Can you work these out from the model? Positions are in its coordinate system, mm. A direction names the side the tool comes from. Coordinates: 2 decimals unless noted, no trailing zeros. Loops run counter-clockwise (first coordinate to the right, second up) from the corner with the lowest first, then second, coordinate; pieces in that order, holes last. Notation, with made-up numbers: (-0.75, 26.5) -> (20.25, 26.5) arc R14 ccw to (20.25, 40.5) -> close; hole circle Ø4 at (75.25, 13). An arc over 180 degrees is marked (long way). Put each result on its own line as item: value. Start each with the question number.
Item 1: We'd pull the mould along X, two halves only. Please class faces 1 (the flat face through (25.4, 614, -25)), 2 (the flat face through (2, 0, -27)), 3 (the flat face through (13, 614, -2.54)): pulls with the +X half, pulls with the -X half, needs draft (parallel to the pull), parting line crosses it, or undercut.
Item 2: Please list where these lines run through material, in increasing order: L1, parallel to Y at x = 1.5, z = -12.7; L2, parallel to Y at x = 1.45, z = -38.1; L3, parallel to X at y = 435, z = -26. Write a range as from..to.
Item 3: For faces 4 (the flat face through (2.54, 614, -25)), 5 (the flat face through (0, 614, -25)), which set-ups out of +Z, -Z, +X, -X, +Y, -Y let a thin tool reach every point of the face, with its end or its side?
Item 4: If we section it at A-A on y = 861: Please give me the cut outline in (x, z).
```python
from build123d import *

# Parameters (mm, degrees)
SKETCH1_W           = 25.4
SKETCH1_H           = 50.8
SKETCH1_W_2         = 20.32
SKETCH1_H_2         = 45.72
EXTRUDE_THIN1_DEPTH = 1244.6
SKETCH2_R           = 2.4892
CUT_EXTRUDE1_DEPTH  = 26.4
SKETCH3_R           = 2.5019
SKETCH3_R_2         = 2.4892
CUT_EXTRUDE2_DEPTH  = 26.4
SKETCH5_R           = 2.4892
CUT_EXTRUDE3_DEPTH  = 51.8
SKETCH6_R           = 3.175
CUT_EXTRUDE4_DEPTH  = 51.8
SKETCH7_R           = 3.175
CUT_EXTRUDE5_DEPTH  = 51.8


with BuildPart() as part:
    # Sketch1 → Extrude-Thin1 (new body)
    with BuildSketch(Plane(origin=(0, 0, 0), x_dir=(1, 0, 0), z_dir=(0, 1, 0))):
        with Locations((12.7, 25.4)):
            Rectangle(SKETCH1_W, SKETCH1_H)
        with Locations((12.7, 25.4)):
            Rectangle(SKETCH1_W_2, SKETCH1_H_2, mode=Mode.SUBTRACT)
    extrude(amount=EXTRUDE_THIN1_DEPTH)

    # Sketch2 → Cut-Extrude1 (cut, through all)
    with BuildSketch(Plane(origin=(25.4, 0, 0), x_dir=(0, 0, -1), z_dir=(1, 0, 0))):
        with Locations((25.4, 1200.15)):
            Circle(SKETCH2_R)
        with Locations((25.4, 1212.85)):
            Circle(SKETCH2_R)
    extrude(amount=-CUT_EXTRUDE1_DEPTH, mode=Mode.SUBTRACT)

    # Sketch3 → Cut-Extrude2 (cut, through all)
    with BuildSketch(Plane.ZY):
        with Locations((-12.7, 721.632068306)):
            Circle(SKETCH3_R)
        with Locations((-38.1, 721.632068306)):
            Circle(SKETCH3_R)
        with Locations((-12.7, 12.960193373)):
            Circle(SKETCH3_R_2)
        with Locations((-38.1, 12.7)):
            Circle(SKETCH3_R_2)
    extrude(amount=-CUT_EXTRUDE2_DEPTH, mode=Mode.SUBTRACT)

    # Sketch5 → Cut-Extrude3 (cut, through all)
    with BuildSketch(Plane(origin=(0, 0, -50.8), x_dir=(-1, 0, 0), z_dir=(0, 0, -1))):
        with Locations((-12.7, 1084.8045868)):
            Circle(SKETCH5_R)
    extrude(amount=-CUT_EXTRUDE3_DEPTH, mode=Mode.SUBTRACT)

    # Sketch6 → Cut-Extrude4 (cut, through all)
    with BuildSketch(Plane(origin=(0, 0, -50.8), x_dir=(-1, 0, 0), z_dir=(0, 0, -1))):
        with Locations((-12.7, 1231.9)):
            Circle(SKETCH6_R)
    extrude(amount=-CUT_EXTRUDE4_DEPTH, mode=Mode.SUBTRACT)

    # Sketch7 → Cut-Extrude5 (cut, through all)
    with BuildSketch(Plane.XY):
        with Locations((7.9375, 1095.9170868)):
            Circle(SKETCH7_R)
        with Locations((17.4625, 1073.6920868)):
            Circle(SKETCH7_R)
    extrude(amount=-CUT_EXTRUDE5_DEPTH, mode=Mode.SUBTRACT)


solid = part.part
```
Solutions:
1. face 1: pulls with the +X half
1. face 2: needs draft
1. face 3: undercut
2. L1: 0..10.47, 15.45..719.13, 724.13..1244.6
2. L2: 0..10.21, 15.19..719.13, 724.13..1244.6
2. L3: 0..2.54, 22.86..25.4
3. face 4: +Y, -Y
3. face 5: +Z, -Z, -X, +Y, -Y
4. outline: (0, -50.8) -> (25.4, -50.8) -> (25.4, 0) -> (0, 0) -> close; hole (2.54, -48.26) -> (22.86, -48.26) -> (22.86, -2.54) -> (2.54, -2.54) -> close
